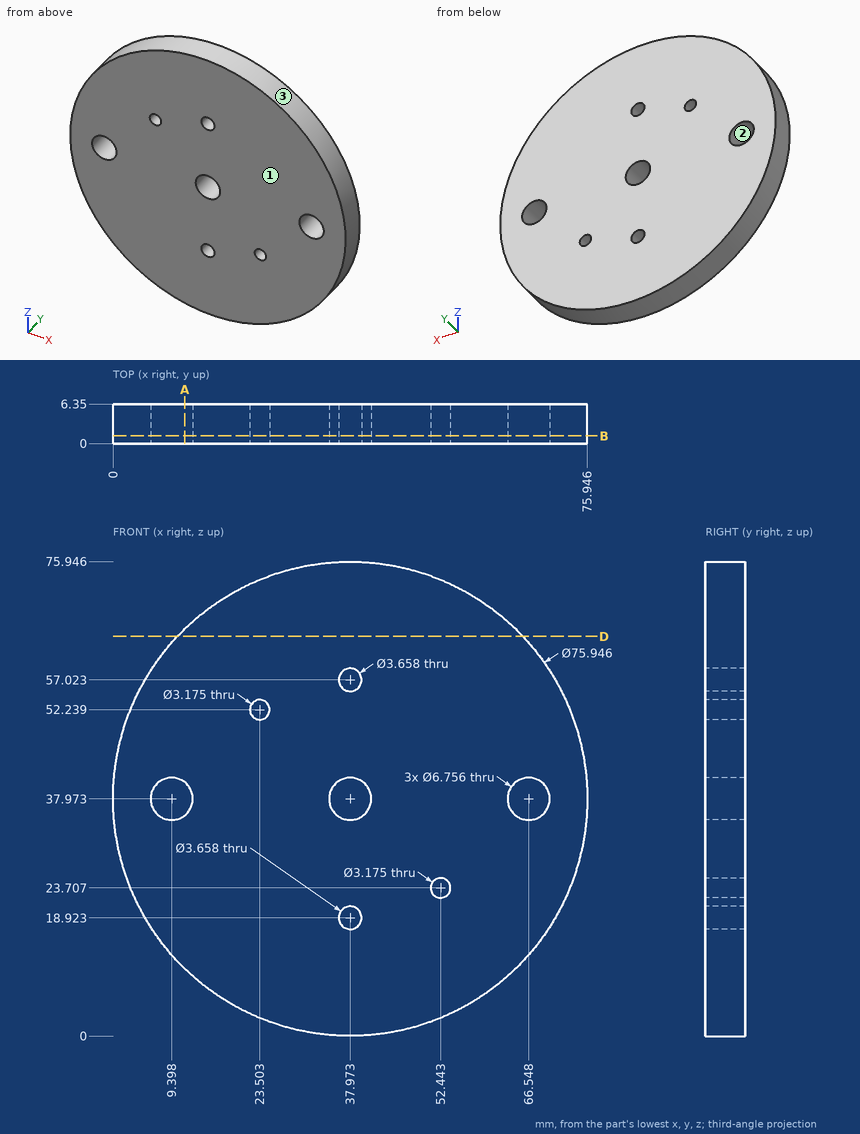
The drawing under review shows one solid part. Ordinate dimensions are in mm from its lowest x, y, z. Coordinates: 2 decimals unless noted, no trailing zeros. Order: outer loops, then holes, each group sorted by start corner. A loop starts at its lowest first (then second) coordinate and runs counter-clockwise, first axis right, second up. Notation, with made-up numbers: (78, 6.5) -> (97, 6.5) arc R21 cw to (97, 13.5) -> close; hole circle Ø10 at (17, -21). An arc over 180 degrees is marked (long way). Use CSV: the item, a comma, the result in double quotes. Start each with the question number.
Item 1: We need section A-A, the plane x = 11.5. Give the boundary of the cut face in (y, z).
Item 2: We need section D-D, the plane z = 64. Give the boundary of the cut face in (x, y), then the cut area to 3 significant figures.
Item 3: We need section B-B, the plane y = 1.25. Give the boundary of the cut face in (x, z) (1 decimal).
Item 4: Insertion check: pin 1 (2 mm diameter, centred on x = 37.973, z = 57.023, fed in from +Y); pin 2 (1.5 mm diameter, centred on x = 12.5, y = 4, fed in from +Z) (1 decimal); pin 3 (1.5 mm diameter, centred on x = 32, y = 4, fed in from +Z) (1 decimal). Each pin has a flat end and moves straight along its axis. Give the tip position at first contact, or say it passes through.
Item 5: Wall thickness on probe 1 along Z at (x, y) = (51, 4) (1 decimal); probe 2 along Z at (x, y) = (63.5, 1) (1 decimal); probe 3 along Z at (x, y) = (39.5, 4.75) (1 decimal): over which ranges is each line inside the solid? List them lowest first.
Item 6: Draft analysis for pull direction X (two halves, no side actions). For the marked faces 1, 2 and 3, state which applies: pulls with the +X half, pulls with the -X half, needs draft (parallel to the pull), parting line crosses it, or undercut.
Derived:
1,outline,"(0, 10.75) -> (6.35, 10.75) -> (6.35, 35.33) -> (0, 35.33) -> close; (0, 40.62) -> (6.35, 40.62) -> (6.35, 65.2) -> (0, 65.2) -> close"
2,outline,"(10.32, 0) -> (65.62, 0) -> (65.62, 6.35) -> (10.32, 6.35) -> close"
2,area,"351 mm^2"
3,outline,"circle Ø75.9 at (38, 38); hole circle Ø6.8 at (9.4, 38); hole circle Ø3.2 at (23.5, 52.2); hole circle Ø6.8 at (38, 38); hole circle Ø3.7 at (38, 18.9); hole circle Ø3.7 at (38, 57); hole circle Ø3.2 at (52.4, 23.7); hole circle Ø6.8 at (66.5, 38)"
4,pin 1,"passes through"
4,pin 2,"stops at z = 66.8"
4,pin 3,"stops at z = 75.6"
5,probe 1,"z = 2.3 to 23, 24.4 to 73.6"
5,probe 2,"z = 9.9 to 36.5, 39.4 to 66.1"
5,probe 3,"z = 0 to 17.9, 19.9 to 35, 41 to 56, 58 to 75.9"
6,face 1,"needs draft"
6,face 2,"undercut"
6,face 3,"parting line crosses it"
